Work out the finished part from the listing and answer in its coordinate system (mm). Face numbers are marked on the shaded views. A direction names the side the tool comes from. Coordinates: 2 decimals unless noted, no trailing zeros. Write each loop counter-clockwise with the first axis right and the second up, starting at its lowest first coordinate (ties: lowest second). Pieces come first, ordered by that corner, then holes. Notation, with made-up numbers: (32, 54.5) - (59, 54.5) arc R4 ccw to (59, 60.5) - close; hole circle Ø1 at (-20.75, 36.25). An arc over 180 degrees is marked (long way). Use one line per item in the form item = value. Start each with the question number.
Item 1: Given pin 1 (4 mm diameter, centred on x = 4, z = -11.5, fed in from +Y); pin 2 (4 mm diameter, centred on x = -12, z = 11, fed in from -Y); pin 3 (4 mm diameter, centred on x = -6.5, y = 349.5, fed in from -Z); pin 4 (6 mm diameter, centred on y = 364, z = -13.5, fed in from +X), each flat-ended and moving along its own axis, determine where each tip first touches the part or whether it passes through.
Item 2: Consider probe 1 along Y at (x, z) = (-8.5, 8); probe 2 along Y at (x, z) = (3, 14.5); probe 3 along Z at (x, y) = (-7, 283.5). Determine where each line is inside the solid, lowest interval first.
Item 3: For the marked faces 4 and 5, determine the directions among +Z, -Z, +X, -X, +Y, -Y from which every point of the face is accessible in a straight line to the end or side of a thin tool.
Item 4: A cutting plane is placed at A-A (y = 286.5). Write down the section's boundary in (x, z).
Item 5: Determine the mould class of the marked faces 1, 2 and 3 for opening direction Y: released by +Y, released by -Y, zero draft, split by the parting line, or undercut.
from build123d import *

# Parameters (mm, degrees)
BOSS_EXTRUDE1_DEPTH   = 7.63
LPATTERN2_COUNT       = 2
LPATTERN2_PITCH       = 53.34
BODY_MOVE_COPY1_ANGLE = 180
LPATTERN3_COUNT       = 3
LPATTERN3_PITCH       = 146.05
BODY_MOVE_COPY2_ANGLE = 120
BODY_MOVE_COPY3_ANGLE = 120
BOSS_EXTRUDE2_START   = -49.53
SKETCH3_R             = 9.5
BOSS_EXTRUDE2_DEPTH   = 466.09


with BuildPart() as part:
    # Sketch1 → Boss-Extrude1 (new body)
    with BuildSketch(Plane(origin=(0, 0, 0), x_dir=(1, 0, 0), z_dir=(0, 1, 0))):
        with BuildLine():
            Line((-5.499261314, 15.875), (-10.998522628, 6.35))
            ThreePointArc((-10.998522628, 6.35), (0, -12.7), (10.998522628, 6.35))
            Line((10.998522628, 6.35), (5.499261314, 15.875))
            ThreePointArc((5.499261314, 15.875), (0, 19.05), (-5.499261314, 15.875))
        make_face()
    extrude(amount=BOSS_EXTRUDE1_DEPTH)


with BuildPart() as lpattern2_1:
    # LPattern2: pattern copy
    add(part.part.moved(Location(Vector(0, 1, 0) * (1 * LPATTERN2_PITCH))))


with BuildPart() as lpattern2_1_1:
    # Body-Move_Copy1: moved
    add(lpattern2_1.part.rotate(Axis((0, 0, 0), (0, 1, 0)), BODY_MOVE_COPY1_ANGLE))


with BuildPart() as lpattern3_1:
    # LPattern3: pattern copy
    add(part.part.moved(Location(Vector(0, 1, 0) * (1 * LPATTERN3_PITCH))))


with BuildPart() as lpattern3_2:
    # LPattern3: pattern copy
    add(part.part.moved(Location(Vector(0, 1, 0) * (2 * LPATTERN3_PITCH))))


with BuildPart() as lpattern3_3:
    # LPattern3: pattern copy
    add(lpattern2_1_1.part.moved(Location(Vector(0, 1, 0) * (1 * LPATTERN3_PITCH))))


with BuildPart() as lpattern3_4:
    # LPattern3: pattern copy
    add(lpattern2_1_1.part.moved(Location(Vector(0, 1, 0) * (2 * LPATTERN3_PITCH))))


with BuildPart() as lpattern3_1_1:
    # Body-Move_Copy2: moved
    add(lpattern3_1.part.rotate(Axis((0, 0, 0), (0, 1, 0)), BODY_MOVE_COPY2_ANGLE))


with BuildPart() as lpattern3_3_1:
    # Body-Move_Copy2: moved
    add(lpattern3_3.part.rotate(Axis((0, 0, 0), (0, 1, 0)), BODY_MOVE_COPY2_ANGLE))


with BuildPart() as lpattern3_2_1:
    # Body-Move_Copy3: moved
    add(lpattern3_2.part.rotate(Axis((0, 0, 0), (0, -1, 0)), BODY_MOVE_COPY3_ANGLE))


with BuildPart() as lpattern3_4_1:
    # Body-Move_Copy3: moved
    add(lpattern3_4.part.rotate(Axis((0, 0, 0), (0, -1, 0)), BODY_MOVE_COPY3_ANGLE))


with BuildPart() as part_1:
    add(part.part)

    add(lpattern2_1_1.part)  # Boss-Extrude2 merges LPattern2_1

    add(lpattern3_1_1.part)  # Boss-Extrude2 merges LPattern3_1

    add(lpattern3_2_1.part)  # Boss-Extrude2 merges LPattern3_2

    add(lpattern3_3_1.part)  # Boss-Extrude2 merges LPattern3_3

    add(lpattern3_4_1.part)  # Boss-Extrude2 merges LPattern3_4
    # Sketch3 → Boss-Extrude2 (add)
    with BuildSketch(Plane(origin=(0, 0, 0), x_dir=(1, 0, 0), z_dir=(0, 1, 0)).offset(BOSS_EXTRUDE2_START)):
        with Locations(Location((0, 0, 0), (0, 0, 270))):
            Circle(SKETCH3_R)
    extrude(amount=BOSS_EXTRUDE2_DEPTH)


solid = part_1.part
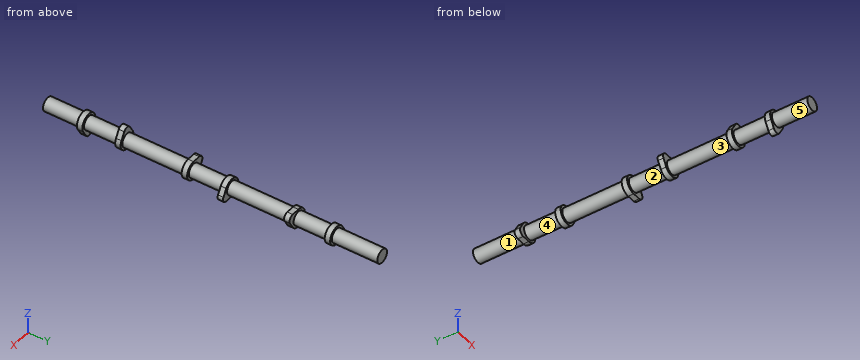
Answer:
q1.pin_1 = 353.07
q1.pin_2 = 146.05
q1.pin_3 = -12.7
q1.pin_4 = through
q2.probe_1 = 0 to 7.63, 53.34 to 60.97, 146.05 to 153.68, 199.39 to 207.02, 292.1 to 299.73, 345.44 to 353.07
q2.probe_2 = 53.34 to 60.97
q2.probe_3 = -6.42 to 6.42
q3.face_4 = none
q3.face_5 = -Y
q4.outline = circle Ø19 at (0, 0)
q5.face_1 = zero draft
q5.face_2 = undercut
q5.face_3 = undercut
